Source: CAD feature listing. Evaluate the final solid. Frame: model axes, mm. Coordinates: 2 decimals unless noted, no trailing zeros. Loops run counter-clockwise (first coordinate to the right, second up) from the corner with the lowest first, then second, coordinate; pieces in that order, holes last. Notation, with made-up numbers: (23.25, 12.25) - (53.25, 12.25) arc R23 cw to (53.25, 26.25) - close; hole circle Ø2 at (74.25, 70). An arc over 180 degrees is marked (long way). Write item = value, one per line. Start each with the question number.
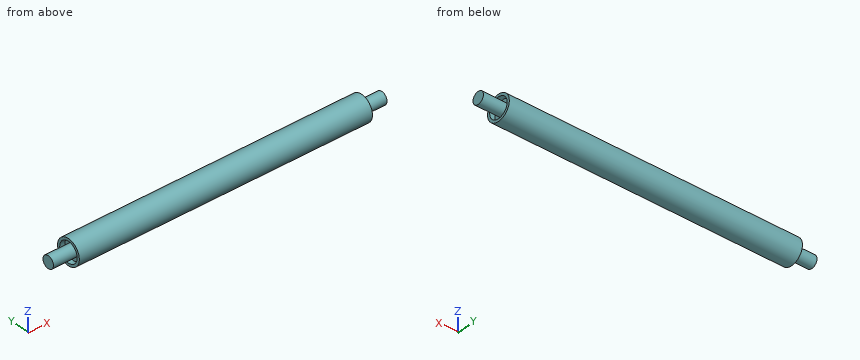
from build123d import *

# Parameters (mm, degrees)
SKETCH_R     = 12.5
PAD_DEPTH    = 145
SKETCH001_R  = 10
POCKET_DEPTH = 5
SKETCH002_R  = 6
PAD001_DEPTH = 25


with BuildPart() as part:
    # Sketch → Pad (new body, symmetric)
    with BuildSketch(Plane.YZ):
        Circle(SKETCH_R)
    extrude(amount=PAD_DEPTH, both=True)

    # Sketch001 (on Face3 of Pad) → Pocket (cut)
    with BuildSketch(Plane.YZ.offset(145)):
        Circle(SKETCH001_R)
    pocket = extrude(amount=-POCKET_DEPTH, mode=Mode.SUBTRACT)

    # Sketch002 (on Face5 of Pocket) → Pad001 (join)
    with BuildSketch(Plane.YZ.offset(140)):
        Circle(SKETCH002_R)
    pad001 = extrude(amount=PAD001_DEPTH)

    # Mirrored: Pocket, Pad001 across YZ
    add(pocket.mirror(Plane.YZ), mode=Mode.SUBTRACT)
    add(pad001.mirror(Plane.YZ))


solid = part.part
Item 1: Material intervals for L1, parallel to Z at x = 143.65, y = 0; L2, parallel to Y at x = 143, z = 5.25; L3, parallel to X at y = 3.75, z = 10.5, sorted ascending. Write a range as [from, to].
Item 2: First-contact query: pin 1 (5 mm diameter, centred on x = -93.5, y = -10, fed in from -Z); pin 2 (2 mm diameter, centred on x = -81, y = 1, fed in from +Z); pin 3 (1 mm diameter, centred on x = 118, y = -2.5, fed in from +Z); pin 4 (3 mm diameter, centred on y = 7, z = -5.5, fed in from -X). Flat tips, straight axial feed; report the tip coordinate or a pass-through.
Item 3: Cut plane A-A (z = 0). Return the cut outline in (x, y), then the cut area to 3 significant figures.
Item 4: Cut plane C-C (x = -20). Return the cut outline in (y, z), then the cut area to 3 significant figures.
Responses:
q1.L1 = [-12.5, -10], [-6, 6], [10, 12.5]
q1.L2 = [-11.34, -8.51], [-2.9, 2.9], [8.51, 11.34]
q1.L3 = [-145, 145]
q2.pin_1 = -10
q2.pin_2 = 12.5
q2.pin_3 = 12.34
q2.pin_4 = -145
q3.outline = (-165, -6) - (-140, -6) - (-140, -10) - (-145, -10) - (-145, -12.5) - (145, -12.5) - (145, -10) - (140, -10) - (140, -6) - (165, -6) - (165, 6) - (140, 6) - (140, 10) - (145, 10) - (145, 12.5) - (-145, 12.5) - (-145, 10) - (-140, 10) - (-140, 6) - (-165, 6) - close
q3.area = 7,650 mm2
q4.outline = circle Ø25 at (0, 0)
q4.area = 491 mm2
